Could you check a few things on this model? Use its own coordinates, in mm. Face numbers are marked on the shaded views. Round coordinates to 2 decimals unless told otherwise and drop trailing zeros. Loops run counter-clockwise (first coordinate to the right, second up) from the corner with the lowest first, then second, coordinate; pieces in that order, holes last. Notation, with made-up numbers: M 5.5,-40 L 42.5,-40 A11 ccw 42.5,-30 Z; hole C 22,-30.75 d10. An arc over 180 degrees is marked long. Answer in a Markdown table with one row per item.
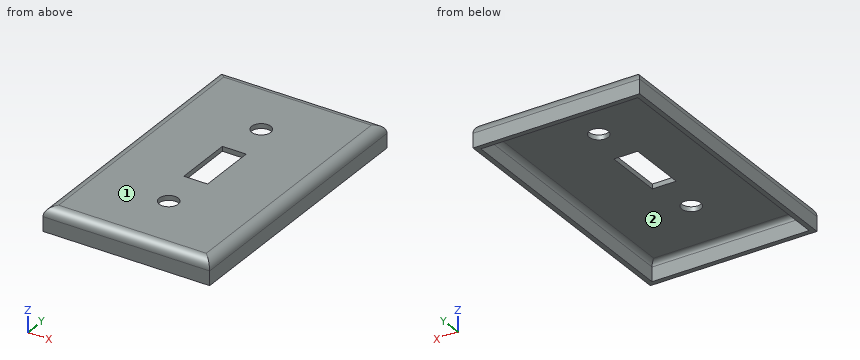
```python
from build123d import *

# Parameters (mm, degrees)
CROQUIS2_W              = 70
CROQUIS2_H              = 115
SALIENTE_EXTRUIR1_DEPTH = 10
REDONDEO1_R             = 4
VACIADO1_T              = -2
CROQUIS3_R              = 4
CROQUIS3_W              = 10
CROQUIS3_H              = 25
CORTAR_EXTRUIR1_DEPTH   = 10


with BuildPart() as part:
    # Croquis2 → Saliente-Extruir1 (new body)
    with BuildSketch(Plane.XY):
        with Locations((35, 57.5)):
            Rectangle(CROQUIS2_W, CROQUIS2_H)
    extrude(amount=SALIENTE_EXTRUIR1_DEPTH)

    # Redondeo1
    redondeo1_edges = [part.edges().sort_by_distance(p)[0] for p in [
        (70, 57.5, 10),
        (35, 115, 10),
        (0, 57.5, 10),
        (35, 0, 10),
    ]]
    fillet(redondeo1_edges, radius=REDONDEO1_R)

    # Vaciado1
    vaciado1_openings = [part.faces().sort_by_distance(p)[0] for p in [
        (35, 57.5, 0),
    ]]
    offset(amount=VACIADO1_T, openings=vaciado1_openings)

    # Croquis3 → Cortar-Extruir1 (cut)
    with BuildSketch(Plane.XY.offset(10)):
        with Locations((35, 87.5)):
            Circle(CROQUIS3_R)
        with Locations((35, 27.5)):
            Circle(CROQUIS3_R)
        with Locations((35, 57.5)):
            Rectangle(CROQUIS3_W, CROQUIS3_H)
    extrude(amount=-CORTAR_EXTRUIR1_DEPTH, mode=Mode.SUBTRACT)


solid = part.part
```
1) Will these pins go through, and if not, where does the flat tip stop? P1, Ø0.6, axis at x = 35.5, z = 9, coming from the -Y side; P2, Ø1, axis at y = 63.5, z = 9.5, coming from the +X side; P3, Ø1.6, axis at x = 33.5, z = 9, coming from the +Y side.
Computed:
| item | result |
|---|---|
| P1 | stops at y = 1.05 |
| P2 | stops at x = 68.65 |
| P3 | stops at y = 114.34 |
2) I want a section at D-D, the plane x = 23. Please give me the cut outline in (y, z).
Computed:
| item | result |
|---|---|
| outline | M 0,0 L 2,0 L 2,6 A2 cw 4,8 L 111,8 A2 cw 113,6 L 113,0 L 115,0 L 115,6 A4 ccw 111,10 L 4,10 A4 ccw 0,6 Z |
3) If we mould it in two halves opening along X, with no side actions, what happens to the marked faces 1 and 2? For each: released by +X, released by -X, zero draft, split by the parting line, or undercut.
Computed:
| item | result |
|---|---|
| face 1 | zero draft |
| face 2 | undercut |
4) I want a section at A-A, the plane y = 48. Please give me the cut outline in (x, z), plus the area to 3 significant figures.
Computed:
| item | result |
|---|---|
| outline | M 0,0 L 2,0 L 2,6 A2 cw 4,8 L 30,8 L 30,10 L 4,10 A4 ccw 0,6 Z; M 40,8 L 66,8 A2 cw 68,6 L 68,0 L 70,0 L 70,6 A4 ccw 66,10 L 40,10 Z |
| area | 147 mm² |
5) I want a section at C-C, the plane y = 107. Please give me the cut outline in (x, z).
Computed:
| item | result |
|---|---|
| outline | M 0,0 L 2,0 L 2,6 A2 cw 4,8 L 66,8 A2 cw 68,6 L 68,0 L 70,0 L 70,6 A4 ccw 66,10 L 4,10 A4 ccw 0,6 Z |
6) I want a section at B-B, the plane x = 35. Please give me the cut outline in (y, z), plus the area to 3 significant figures.
Computed:
| item | result |
|---|---|
| outline | M 0,0 L 2,0 L 2,6 A2 cw 4,8 L 23.5,8 L 23.5,10 L 4,10 A4 ccw 0,6 Z; M 31.5,8 L 45,8 L 45,10 L 31.5,10 Z; M 70,8 L 83.5,8 L 83.5,10 L 70,10 Z; M 91.5,8 L 111,8 A2 cw 113,6 L 113,0 L 115,0 L 115,6 A4 ccw 111,10 L 91.5,10 Z |
| area | 175 mm² |
7) I need wall thicknesses on line 1 (Y direction, x = 35, z = 8.6); line 2 (Y direction, x = 58.5, z = 4); line 3 (Y direction, x = 35, z = 9.6). Which ranges of each line are inside material? Lowest first, please.
Computed:
| item | result |
|---|---|
| line 1 | y = 0.96 to 23.5, 31.5 to 45, 70 to 83.5, 91.5 to 114.04 |
| line 2 | y = 0 to 2, 113 to 115 |
| line 3 | y = 2.26 to 23.5, 31.5 to 45, 70 to 83.5, 91.5 to 112.74 |
